Autodesk Inventor part; units mm, degrees
ref_plane "YZ Plane" through (0, 0, 0) normal (1, 0, 0) x (0, 1, 0)
ref_plane "XZ Plane" through (0, 0, 0) normal (0, 1, 0) x (-1, 0, 0)
ref_plane "XY Plane" through (0, 0, 0) normal (0, 0, 1) x (1, 0, 0)
sketch "Sketch1" plane through (0, 0, 0) normal (0, 0, 1) x (1, 0, 0)
  line L0 (-50.984, -65) -> (50.984, -65)
  line L1 (50.984, -65) -> (50.984, 65)
  line L2 (50.984, 65) -> (-50.984, 65)
  line L3 (-50.984, 65) -> (-50.984, -65)
  line L4 (-50.984, -65) -> (50.984, 65) construction
  line L5 (50.984, -65) -> (-50.984, 65) construction
  line L6 (-55.984, 70) -> (55.984, 70)
  line L7 (55.984, 70) -> (55.984, -70)
  line L8 (55.984, -70) -> (-55.984, -70)
  line L9 (-55.984, -70) -> (-55.984, 70)
  point P0 (0, 0)
  dimension "d0" = 101.968
  dimension "d1" = 130
  dimension "d2" = 5
extrude "Extrusion1" add sketch "Sketch1" along normal blind 50
sketch "Sketch5" plane through (50.984, -65, 0) normal (-1, 0, 0) x (0, 0, 1)
  line L0 (0, -5) -> (50, -5)
  line L1 (0, 135) -> (50, 135)
  circle A0 centre (25, 65) radius 12
  line L2 (50, 135) -> (50, -5)
  point P0 (0, 65)
  dimension "d14" = 140
  dimension "d15" = 24
  dimension "d16" = 25
  dimension "d17" = 70
extrude "Extrusion5" cut sketch "Sketch5" against normal blind 2.778
sketch "Sketch6" plane through (55.984, -70, 0) normal (1, 0, 0) x (0, 0, -1)
  line L0 (0, 0) -> (0, 140)
  line L1 (0, 140) -> (-50, 140)
  line L2 (-50, 0) -> (-50, 140)
  line L3 (0, 0) -> (-50, 0)
  point P0 (0, 70)
extrude "Extrusion6" add sketch "Sketch6" along normal blind 2.778
sketch "Sketch8" plane through (0, 0, 0) normal (0, 0, -1) x (-1, 0, 0)
  line L0 (55.984, -70) -> (-58.762, -70)
  line L1 (55.984, 70) -> (55.984, -70)
  line L2 (55.984, 70) -> (-58.762, 70)
  line L3 (-58.762, -70) -> (-58.762, 70)
  line L4 (50.984, -65) -> (50.984, 65)
  line L5 (-50.984, -65) -> (50.984, -65)
  line L6 (-50.984, 65) -> (-50.984, -65)
  line L7 (50.984, 65) -> (-50.984, 65)
  point P0 (0, 0)
extrude "Extrusion8" add sketch "Sketch8" along normal blind 17.5
sketch "Sketch9" plane through (0, 0, 50) normal (0, 0, 1) x (1, 0, 0)
  line L0 (-55.984, -70) -> (58.762, -70)
  line L1 (58.762, 70) -> (58.762, -70)
  line L2 (-55.984, 70) -> (58.762, 70)
  line L3 (-55.984, 70) -> (-55.984, -70)
  line L4 (-50.984, -65) -> (-50.984, 65)
  line L5 (-50.984, 65) -> (50.984, 65)
  line L6 (50.984, 65) -> (50.984, -65)
  line L7 (50.984, -65) -> (-50.984, -65)
  point P0 (0, 0)
extrude "Extrusion9" add sketch "Sketch9" along normal blind 17.5
fillet "Fillet1" radius 8 1 edges at (-50.984, -65, 25)
fillet "Fillet2" radius 8 3 edges at (50.984, -65, 25) (50.984, 65, 25) (-50.984, 65, 25)
sketch "Sketch10" plane through (-55.984, -70, -17.5) normal (-1, 0, 0) x (0, 0, 1)
  circle A0 centre (42.5, 70) radius 6.25
  circle A1 centre (37.767, 78.237) radius 1.65
  line L0 (0, 0) -> (0, 140)
  line L1 (85, 0) -> (0, 0)
  circle A2 centre (37.733, 61.7537) radius 1.65
  circle A3 centre (49.5, 85.5) radius 1.65
  circle A4 centre (49.5, 54.5) radius 1.65
  circle A5 centre (62.923, 77.75) radius 1.65
  circle A6 centre (62.923, 62.25) radius 1.65
  point P0 (17.5, 70)
  dimension "d31" = 12.5
  dimension "d32" = 3.3
  dimension "d33" = 37.767
  dimension "d34" = 78.237
  dimension "d35" = 3.3
  dimension "d36" = 37.733
  dimension "d38" = 61.7537
  dimension "d39" = 3.3
  dimension "d41" = 85.5
  dimension "d42" = 49.5
  dimension "d43" = 3.3
  dimension "d44" = 54.5
  dimension "d45" = 3.3
  dimension "d46" = 77.75
  dimension "d47" = 62.923
  dimension "d48" = 3.3
  dimension "d49" = 62.25
  dimension "d50" = 62.923
extrude "Extrusion10" cut sketch "Sketch10" against normal blind 5
sketch "Sketch11" plane through (-55.984, -70, -17.5) normal (-1, 0, 0) x (0, 0, 1)
  circle A0 centre (42.5, 21.5) radius 3.25
  circle A1 centre (42.5, 118.5) radius 3.25
  line L0 (0, 140) -> (85, 140)
  line L1 (85, 0) -> (0, 0)
  point P0 (17.5, 70)
  dimension "d53" = 6.5
  dimension "d54" = 6.5
  dimension "d58" = 21.5
  dimension "d59" = 21.5
extrude "Extrusion12" cut sketch "Sketch11" against normal blind 10
sketch "Sketch12" plane through (-55.984, -70, -17.5) normal (0, -1, 0) x (1, 0, 0)
  circle A0 centre (21.5, 42.5) radius 3.25
  line L0 (0, 85) -> (0, 0)
  point P0 (55.984, 17.5)
  dimension "d62" = 6.5
  dimension "d63" = 21.5
sketch "Sketch13" plane through (-55.984, 70, -17.5) normal (0, 1, 0) x (1, 0, 0)
  circle A0 centre (21.5, -42.5) radius 3.25
  line L0 (0, 0) -> (0, -85)
  point P0 (55.984, -17.5)
  dimension "d66" = 6.5
  dimension "d67" = 21.5
extrude "Extrusion13" cut sketch "Sketch12" against normal blind 10
extrude "Extrusion14" cut sketch "Sketch13" against normal blind 10
properties part number "caja conexion"
Input: part model. Units: mm. Frame: model coordinates. A direction names the side the tool comes from. Round coordinates to 2 decimals unless told otherwise and drop trailing zeros. Loops run counter-clockwise (first coordinate to the right, second up) from the corner with the lowest first, then second, coordinate; pieces in that order, holes last.
1) Section query B-B on x = 19. Return the cut outline in (y, z).
Ans:
outline: (-70, -17.5) - (-65, -17.5) - (-65, 67.5) - (-70, 67.5) - close; (65, -17.5) - (70, -17.5) - (70, 67.5) - (65, 67.5) - close
2) Material intervals for line 1 (Y direction, x = -26.5, z = 32.5); line 2 (X direction, y = 2, z = 44.5); line 3 (Y direction, x = 53, z = 25), sorted ascending.
Ans:
line 1: y = -70 to -65, 65 to 70
line 2: x = -55.98 to -50.98, 50.98 to 58.76
line 3: y = -70 to -12, 12 to 70
3) Set-up query: faces 1 (the flat face through (-1, 65, 24)), 2 (the flat face through (1, -70, 24)), 3 (the flat face through (53.762, 0, 25)), 4 (the cylindrical face through (-53.519, -9.25, 18.924)), 5 (the flat face through (58.762, 1, 24)). Return all of +Z, -Z, +X, -X, +Y, -Y with unobstructed straight access to the full face (end or side cutting, diameter ignored); none if empty.
Ans:
face 1: +Z, -Z
face 2: +Z, -Z, +X, -X, -Y
face 3: none
face 4: -X
face 5: +Z, -Z, +X, +Y, -Y
4) Pin query (flat end, axial travel): pin 1 (2 mm diameter, centred on y = 7.75, z = 45.423, fed in from -X); pin 2 (4 mm diameter, centred on y = -8.25, z = 20.23, fed in from -X); pin 3 (4 mm diameter, centred on x = -34.484, z = 25, fed in from +Y). Return the tip coordinate at first contact, or that it passes through.
Ans:
pin 1: stops at x = 50.98
pin 2: stops at x = -55.98
pin 3: passes through
5) Pull-direction query (Z, two-part tool) for faces 6 (the flat face through (-55.984, 1, 15)), 7 (the cylindrical face through (-31.48, 67.54, 26.24)), 8 (the cylindrical face through (-53.52, -8.38, 46.95)), 9 (the flat face through (52, 0, 67.5)); classes: released by +Z, released by -Z, zero draft, split by the parting line, or undercut.
Ans:
face 6: zero draft
face 7: undercut
face 8: undercut
face 9: released by +Z
6) Section query C-C on y = -41.5. Return the cut outline in (x, z).
Ans:
outline: (-55.98, -17.5) - (-50.98, -17.5) - (-50.98, 67.5) - (-55.98, 67.5) - close; (50.98, -17.5) - (58.76, -17.5) - (58.76, 67.5) - (50.98, 67.5) - close
7) Section query D-D on z = -1.5. Return the cut outline in (x, y), plus the area to 3 significant figures.
Ans:
outline: (-55.98, -70) - (58.76, -70) - (58.76, 70) - (-55.98, 70) - close; hole (-50.98, -57) arc R8 ccw to (-42.98, -65) - (42.98, -65) arc R8 ccw to (50.98, -57) - (50.98, 57) arc R8 ccw to (42.98, 65) - (-42.98, 65) arc R8 ccw to (-50.98, 57) - close
area: 2,860 mm2
8) Section query A-A on y = 0. Return the cut outline in (x, z), plus the area to 3 significant figures.
Ans:
outline: (-55.98, -17.5) - (-50.98, -17.5) - (-50.98, 18.75) - (-55.98, 18.75) - close; (-55.98, 31.25) - (-50.98, 31.25) - (-50.98, 67.5) - (-55.98, 67.5) - close; (50.98, -17.5) - (58.76, -17.5) - (58.76, 67.5) - (50.98, 67.5) - (50.98, 37) - (53.76, 37) - (53.76, 13) - (50.98, 13) - close
area: 957 mm2
